```python
from build123d import *

# Parameters (mm, degrees)
F1_DEPTH    = 4
F2_T4_DEPTH = 24
F3_T4_DEPTH = 19
F4_T4_DEPTH = 14
F5_R        = 0.99999
F7_DEPTH    = 25


# Not quite as in the source:
# - a fillet or chamfer that OpenCascade refuses, or shapes differently, is made with other operations: its cross-section is extruded or revolved along the edge and cut away or added
# - a fillet or chamfer is up to 0.001 mm smaller than in the source, because OpenCascade refuses the exact size


with BuildPart() as f1:
    # F0 (on Top) → F1 (new body)
    with BuildSketch(Plane.XY):
        Polygon((4, 0), (5, 0), (5, 1), (4, 1), (4, 2), (2, 2), (2, 3), (-1, 3), (-1, 4), (-5, 4), (-5, 0), align=None)
        Polygon((-14, 0), (-5, 0), (-5, 4), (-9, 4), (-9, 3), (-12, 3), (-12, 2), (-14, 2), (-14, 1), (-15, 1), (-15, 0), align=None)
    extrude(amount=F1_DEPTH)

    # F2: fillet of radius 4 on 1 edges, made by hand


with BuildPart() as f2_tool2:
    # F2_s3 → F2_t4 (new body)
    with BuildSketch(Plane.XY.offset(-10)):
        with BuildLine():
            ThreePointArc((-5, 4), (-7.8284271247, 2.8284271247), (-9, 0))
            Line((-9, 0), (-9, 4))
            Line((-9, 4), (-5, 4))
        make_face()
    extrude(amount=F2_T4_DEPTH)

    split(bisect_by=Plane.XZ.offset(-3), keep=Keep.BOTTOM)


with BuildPart() as f1_1:
    add(f1.part)

    # F2_t1: cut F2_tool2
    add(f2_tool2.part, mode=Mode.SUBTRACT)

    # F3: fillet of radius 3 on 1 edges, made by hand


with BuildPart() as f3_tool2:
    # F3_s3 → F3_t4 (new body)
    with BuildSketch(Plane.XY.offset(-7.5)):
        with BuildLine():
            ThreePointArc((-12, 0), (-11.1213203436, 2.1213203436), (-9, 3))
            Line((-9, 3), (-12, 3))
            Line((-12, 3), (-12, 0))
        make_face()
    extrude(amount=F3_T4_DEPTH)

    split(bisect_by=Plane.XZ.offset(-2), keep=Keep.BOTTOM)


with BuildPart() as f1_2:
    add(f1_1.part)

    # F3_t1: cut F3_tool2
    add(f3_tool2.part, mode=Mode.SUBTRACT)

    # F4: fillet of radius 2 on 1 edges, made by hand


with BuildPart() as f4_tool2:
    # F4_s3 → F4_t4 (new body)
    with BuildSketch(Plane.XY.offset(-5)):
        with BuildLine():
            ThreePointArc((-14, 0), (-13.4142135624, 1.4142135624), (-12, 2))
            Line((-12, 2), (-14, 2))
            Line((-14, 2), (-14, 0))
        make_face()
    extrude(amount=F4_T4_DEPTH)

    split(bisect_by=Plane.XZ.offset(-1), keep=Keep.BOTTOM)


with BuildPart() as f1_3:
    add(f1_2.part)

    # F4_t1: cut F4_tool2
    add(f4_tool2.part, mode=Mode.SUBTRACT)

    # F5 (radius 1 in the source; OpenCascade refuses exactly that, so slightly less here)
    f5_edges = [f1_3.edges().sort_by_distance(p)[0] for p in [
        (-15, 1, 2),
    ]]
    fillet(f5_edges, radius=F5_R)

    # F6 (on face) → F7 (intersect)
    with BuildSketch(Plane.XZ):
        Polygon((-5, 0), (5, 0), (5, 1), (4, 1), (4, 2), (2, 2), (2, 3), (-1, 3), (-1, 4), (-5, 4), align=None)
    extrude(amount=-F7_DEPTH, mode=Mode.INTERSECT)


solid = f1_3.part
```
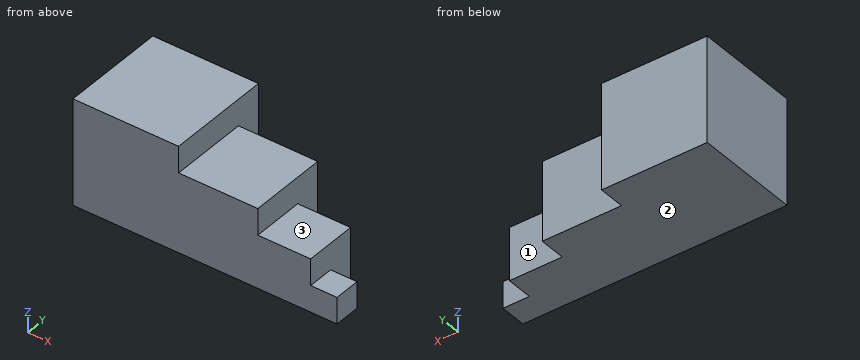
Source: CAD feature listing. Evaluate the final solid. Frame: model axes, mm. Face numbers are marked on the shaded views. A direction names the side the tool comes from. Coordinates: 2 decimals unless noted, no trailing zeros. Order: outer loops, then holes, each group sorted by start corner. A loop starts at its lowest first (then second) coordinate and runs counter-clockwise, first axis right, second up. Notation, with made-up numbers: M 84,1.5 L 106,1.5 A32 ccw 106,39.5 Z; hole C -27.75,-2.5 d9. An arc over 180 degrees is marked long. Write each question's results on one line, items separated by ' | '. Start each with the question number.
1) Access query for the marked faces 1, 2 and 3. Directions: +Z, -Z, +X, -X, +Y, -Y. A direction counts if a zero-diameter tool reaches every point of the face in a straight line with its end or side. Return the directions, or none.
2) Line query: line 1 (X direction, y = 3.7, z = 3.5); line 2 (Y direction, x = 0, z = 2.8); line 3 (X direction, y = 2.65, z = 1.85). Output: solid intervals per line, ascending. Write a range as from..to.
3) Section query B-B (x = 2.5). Return the cut outline in (y, z).
4) Section query A-A (y = 2.55). Return the cut outline in (x, z).
5) Section query D-D (y = 1.9). Return the cut outline in (x, z), plus the area to 3 significant figures.
6) Contact query for flat-ended pins moving along their axis: pin 1 Ø1.6 at (x, y) = (3.5, 1) entering from +Z; pin 2 Ø1.5 at (x, y) = (0.5, 1) entering from +Z; pin 3 Ø0.5 at (x, y) = (4.5, 0.5) entering from +Z. Output: stop coordinate, or through.
Answers:
1) face 1: +Z, -Z, +X, +Y | face 2: -Z, +X, -X, +Y, -Y | face 3: +Z, +X, +Y, -Y
2) line 1: x = -5..-1 | line 2: y = 0..3 | line 3: x = -5..2
3) outline: M 0,0 L 2,0 L 2,2 L 0,2 Z
4) outline: M -5,0 L 2,0 L 2,3 L -1,3 L -1,4 L -5,4 Z
5) outline: M -5,0 L 4,0 L 4,2 L 2,2 L 2,3 L -1,3 L -1,4 L -5,4 Z | area: 29.0 mm^2
6) pin 1: stops at z = 2 | pin 2: stops at z = 3 | pin 3: stops at z = 1
